```python
from build123d import *

# Parameters (mm, degrees)
SKETCH1_W          = 20
SKETCH1_H          = 16.5
SKETCH1_W_2        = 14.6
SKETCH1_H_2        = 13.85
SKETCH1_W_3        = 3
SKETCH1_H_3        = 1
SKETCH1_W_4        = 3.3
SKETCH1_H_4        = 1.15
SKETCH3_W          = 10.5
SKETCH3_H          = 2.5
CUT_EXTRUDE1_DEPTH = 8


with BuildPart() as part:
    # Sketch1 → Revolve1 (revolve)
    with BuildSketch(Plane.XY):
        with Locations((10, 8.25)):
            Rectangle(SKETCH1_W, SKETCH1_H)
        with Locations((27.3, 6.925)):
            Rectangle(SKETCH1_W_2, SKETCH1_H_2)
        with Locations((36.1, 6.925)):
            Rectangle(SKETCH1_W_3, SKETCH1_H_2)
        with Locations((36.1, 14.35)):
            Rectangle(SKETCH1_W_3, SKETCH1_H_3)
        Polygon((37.6, 13.85), (37.6, 0), (52.6, 0), (52.6, 5), (52.6, 13.85), align=None)
        Polygon((52.6, 5), (52.6, 0), (54.8, 0), (54.8, 1.15), (54.8, 5), align=None)
        with Locations((56.45, 0.575)):
            Rectangle(SKETCH1_W_4, SKETCH1_H_4)
    revolve(axis=Axis((0, 0, 0), (1, 0, 0)))

    # Sketch3 → Revolve2 (revolve)
    with BuildSketch(Plane.XY):
        with Locations((-7.25, 7.25)):
            Rectangle(SKETCH3_W, SKETCH3_H)
        Polygon((-2, 8.5), (-2, 6), (0, 6), (0, 11), (-2, 11), align=None)
    revolve(axis=Axis((-12.5, 6, 0), (1, 0, 0)))

    # Sketch4 → Cut-Extrude1 (cut)
    with BuildSketch(Plane.ZY.offset(12.5)):
        Polygon((-72.605280298, 7.5), (-2, 7.5), (2, 7.5), (72.605280298, 7.5), (72.605280298, 148.710560596), (-72.605280298, 148.710560596), align=None)
    extrude(amount=-CUT_EXTRUDE1_DEPTH, mode=Mode.SUBTRACT)


solid = part.part
```
Geometry check sheet. Reference: the model listing, model coordinates, mm. A direction names the side the tool comes from. Coordinates: 2 decimals unless noted, no trailing zeros. Order: outer loops, then holes, each group sorted by start corner. A loop starts at its lowest first (then second) coordinate and runs counter-clockwise, first axis right, second up. Notation, with made-up numbers: (51, 66.25) - (58, 66.25) arc R11 cw to (58, 70.25) - close; hole circle Ø6 at (62.5, 25). An arc over 180 degrees is marked (long way). Answer in a Markdown table with one row per item. Add a question column.
1. Section check D-D (y = 13). Enter the section's corners in (x, z).
2. Material ranges on L1, parallel to X at y = -14.5, z = 2.5; L2, parallel to X at y = 3.5, z = -1.5; L3, parallel to X at y = 10, z = 12.5, recorded low to high. Write a range as [from, to].
3. Section check C-C (x = 6.5). Enter the section's corners in (y, z), plus the area to 3 significant figures.
4. Access from +Z, -Z, +X, -X, +Y, -Y to the whole of each face (thin tool, end or side, straight path). Record for faces 1 (the face through (52.6, -6, 0)), 2 (the face through (27.2, 13.21, 4.16)), 3 (the face through (-9, 7.5, 0)), 4 (the face through (-1, 2, -3)).
5. Section check B-B (y = 0). Enter the section's corners in (x, z), plus the area to 3 significant figures.
6. Gauge pin test, flat ends, axial feed: pin 1 Ø12 at (x, z) = (43, -9.5) entering from -Y; pin 2 Ø5 at (x, y) = (35, -12.5) entering from -Z; pin 3 Ø5 at (x, y) = (31.5, -12.5) entering from +Z. Record the tip position at first contact, or that the pin passes through.
Data:
| question | item | result |
|---|---|---|
| 1 | outline | (0, -10.16) - (20, -10.16) - (20, -4.78) - (34.6, -4.78) - (34.6, -7.18) - (37.6, -7.18) - (37.6, -4.78) - (52.6, -4.78) - (52.6, 4.78) - (37.6, 4.78) - (37.6, 7.18) - (34.6, 7.18) - (34.6, 4.78) - (20, 4.78) - (20, 10.16) - (0, 10.16) - close |
| 2 | L1 | x = [0, 20], [34.6, 37.6] |
| 2 | L2 | x = [-2, 54.8] |
| 2 | L3 | x = [0, 20] |
| 3 | outline | circle Ø33 at (0, 0) |
| 3 | area | 855 mm² |
| 4 | face 1 | +X |
| 4 | face 2 | none |
| 4 | face 3 | +Z, -Z, -X, +Y |
| 4 | face 4 | -X |
| 5 | outline | (0, -16.5) - (20, -16.5) - (20, -13.85) - (34.6, -13.85) - (34.6, -14.85) - (37.6, -14.85) - (37.6, -13.85) - (52.6, -13.85) - (52.6, -5) - (54.8, -5) - (54.8, -1.15) - (58.1, -1.15) - (58.1, 1.15) - (54.8, 1.15) - (54.8, 5) - (52.6, 5) - (52.6, 13.85) - (37.6, 13.85) - (37.6, 14.85) - (34.6, 14.85) - (34.6, 13.85) - (20, 13.85) - (20, 16.5) - (0, 16.5) - close |
| 5 | area | 1,600 mm² |
| 6 | pin 1 | stops at y = -13.4 |
| 6 | pin 2 | stops at z = -10.98 |
| 6 | pin 3 | stops at z = 9.58 |
